The listing builds one solid part. Answer for the finished solid, in the listing's coordinates (mm). Face numbers are marked on the shaded views. A direction names the side the tool comes from. Round coordinates to 2 decimals unless told otherwise and drop trailing zeros. Order: outer loops, then holes, each group sorted by start corner. A loop starts at its lowest first (then second) coordinate and runs counter-clockwise, first axis right, second up. Notation, with made-up numbers: (-5.5, 5.25) -> (1.5, 5.25) arc R26 ccw to (1.5, 41.25) -> close; hole circle Ø11 at (-10, 42). An arc over 180 degrees is marked (long way). Answer in a Markdown table with one row per item. Add a question column.
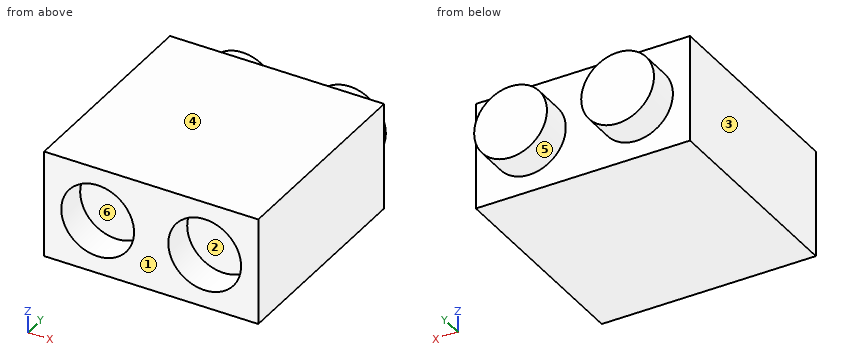
Autodesk Inventor part; units mm, degrees
ref_plane "YZ Plane" through (0, 0, 0) normal (1, 0, 0) x (0, 1, 0)
ref_plane "XZ Plane" through (0, 0, 0) normal (0, 1, 0) x (-1, 0, 0)
ref_plane "XY Plane" through (0, 0, 0) normal (0, 0, 1) x (1, 0, 0)
sketch "草圖2" plane through (0, 0, 0) normal (0, 1, 0) x (-1, 0, 0)
  line L0 (5, 2.5) -> (-5, 2.5)
  line L1 (-5, 2.5) -> (-5, -2.5)
  line L2 (-5, -2.5) -> (5, -2.5)
  line L3 (5, -2.5) -> (5, 2.5)
  circle A0 centre (2.5, 0) radius 1.7
  circle A1 centre (-2.5, 0) radius 1.7
  point P0 (0, 0)
  point P1 (5, 0)
  point P2 (0, -2.5)
  dimension "d0" = 10
  dimension "d1" = 5
  dimension "d2" = 3.4
  dimension "d3" = 2.5
  dimension "d4" = 2.5
  dimension "d7" = 5
extrude "擠出1" add sketch "草圖2" along normal blind 10 contours L3 L2 L1 L0 | A0 | A1
extrude "擠出2" cut sketch "草圖2" along normal blind 1.5 contours A0 | A1
sketch "草圖3" plane through (0, 10, 0) normal (0, 1, 0) x (1, 0, 0)
  circle A0 centre (-2.5, 0) radius 1.7
  circle A1 centre (2.5, 0) radius 1.7
  point P0 (0, 0)
extrude "擠出3" add sketch "草圖3" along normal blind 1.5
sketch "草圖4" plane through (0, 0, 0) normal (0, 0, 1) x (1, 0, 0)
  line L0 (5, 10) -> (5, 0)
  line L1 (5, 0) -> (4.2, 0)
  line L2 (4.2, 0) -> (4.2, 1.5)
  line L3 (4.2, 1.5) -> (0.8, 1.5)
  line L4 (0.8, 1.5) -> (0.8, 0)
  line L5 (0.8, 0) -> (-0.8, 0)
  line L6 (-0.8, 0) -> (-0.8, 1.5)
  line L7 (-0.8, 1.5) -> (-4.2, 1.5)
  line L8 (-4.2, 1.5) -> (-4.2, 0)
  line L9 (-4.2, 0) -> (-5, 0)
  line L10 (-5, 0) -> (-5, 10)
  line L11 (-5, 10) -> (-4.2, 10)
  line L12 (-4.2, 10) -> (-4.2, 11.5)
  line L13 (-4.2, 11.5) -> (-0.8, 11.5)
  line L14 (-0.8, 11.5) -> (-0.8, 10)
  line L15 (-0.8, 10) -> (0.8, 10)
  line L16 (0.8, 10) -> (0.8, 11.5)
  line L17 (0.8, 11.5) -> (4.2, 11.5)
  line L18 (4.2, 11.5) -> (4.2, 10)
  line L19 (4.2, 10) -> (5, 10)
  line L20 (-3, 8) -> (3, 8)
  line L21 (3, 8) -> (3, 2)
  line L22 (3, 2) -> (-3, 2)
  line L23 (-3, 2) -> (-3, 8)
  line L24 (0, 10) -> (0, 0) construction
  line L25 (5, 0) -> (-5, 0) construction
  point P0 (0, 8)
  point P1 (3, 5)
  point P2 (5, 5)
  dimension "d18" = 6
  dimension "d19" = 6
split_face "分割1"
properties part number "110033226_ipt_22_塔樓牆壁"
Item 1: The part is cut by section A-A, the plane x = 2.5. Give the vertices of the cut face in (y, z), and give its area (3 significant figures).
Item 2: Find the intervals of material crossed by probe 1 along Z at (x, y) = (2.5, 0.65); probe 2 along Y at (x, z) = (-3.75, 0.45); probe 3 along Y at (x, z) = (2, -1.7), in increasing order. Write a range as [from, to].
Item 3: The part is cut by section B-B, the plane z = 0.5. Give the vertices of the cut face in (x, y).
Item 4: A tool of negligible diameter and unlimited length cuts with its end or side. For the marked faces 4, 5 and 6, from which of +Z, -Z, +X, -X, +Y, -Y can it reach the whole face along a straight path? Write none if from no direction.
Item 5: For a pull along X with two mould halves and no side action, classify the marked faces 1, 2 and 3 as released by +X, released by -X, zero draft, split by the parting line, or undercut.
Resolved:
| question | item | result |
|---|---|---|
| 1 | outline | (0, -2.5) -> (10, -2.5) -> (10, -1.7) -> (11.5, -1.7) -> (11.5, 1.7) -> (10, 1.7) -> (10, 2.5) -> (0, 2.5) -> (0, 1.7) -> (1.5, 1.7) -> (1.5, -1.7) -> (0, -1.7) -> close |
| 1 | area | 50.0 mm2 |
| 2 | probe 1 | [-2.5, -1.7], [1.7, 2.5] |
| 2 | probe 2 | [1.5, 11.5] |
| 2 | probe 3 | [0, 10] |
| 3 | outline | (-5, 0) -> (-4.12, 0) -> (-4.12, 1.5) -> (-0.88, 1.5) -> (-0.88, 0) -> (0.88, 0) -> (0.88, 1.5) -> (4.12, 1.5) -> (4.12, 0) -> (5, 0) -> (5, 10) -> (4.12, 10) -> (4.12, 11.5) -> (0.88, 11.5) -> (0.88, 10) -> (-0.88, 10) -> (-0.88, 11.5) -> (-4.12, 11.5) -> (-4.12, 10) -> (-5, 10) -> close |
| 4 | face 4 | +Z, +X, -X, +Y, -Y |
| 4 | face 5 | +Y |
| 4 | face 6 | -Y |
| 5 | face 1 | zero draft |
| 5 | face 2 | undercut |
| 5 | face 3 | released by -X |
